Design review of the part built by this model. Coordinates are the model's own, in mm. Face numbers are marked on the shaded views. A direction names the side the tool comes from. Give positions to 0.01 mm unless a question says otherwise; leave off trailing zeros. Loops run counter-clockwise (first coordinate to the right, second up) from the corner with the lowest first, then second, coordinate; pieces in that order, holes last. Notation, with made-up numbers: M 3.25,-14 L 53.25,-14 A5 cw 53.25,-10 Z; hole C -7.75,88.5 d7. An arc over 180 degrees is marked long. Use a Markdown table: item, result. Add a question column.
(1) For the marked faces 1 and 2, list the 3-axis set-ups (+Z, -Z, +X, -X, +Y, -Y) from which the entire face can be reached by the end or side of a thin tool; tool diameter is ignored.
(2) Draft analysis for pull direction X (two halves, no side actions). For the marked faces 3, 4 and 5, state which applies: pulls with the +X half, pulls with the -X half, needs draft (parallel to the pull), parting line crosses it, or undercut.
(3) Add section A-A, the plane x = 1.25. Give the boundary of the cut face in (y, z).
(4) For probe 1 along Z at (x, y) = (2.25, 0); probe 2 along Y at (x, z) = (-4.5, 0); probe 3 along X at (y, z) = (5.75, -118.5), list the stretches that pass through material, from the lowest coordinate up.
(5) Add section B-B, the plane z = -104. Give the boundary of the cut face in (x, y).
(6) Add section C-C, the plane y = -7.5. Give the boundary of the cut face in (x, z), then the cut area to 3 significant figures.
(7) Add section D-D, the plane x = 10.75. Give the boundary of the cut face in (y, z).
(8) Insertion check: pin 1 Ø2 at (x, y) = (-10, -0.5) entering from -Z; pin 2 Ø2 at (x, y) = (5, 0.5) entering from -Z; pin 3 Ø5 at (x, y) = (-9, 8) entering from +Z (3 decimals); pin 4 Ø2 at (x, y) = (1, 8.5) entering from -Z. Each pin has a flat end and moves straight along its axis. Give the tip position at first contact, or say it passes through.
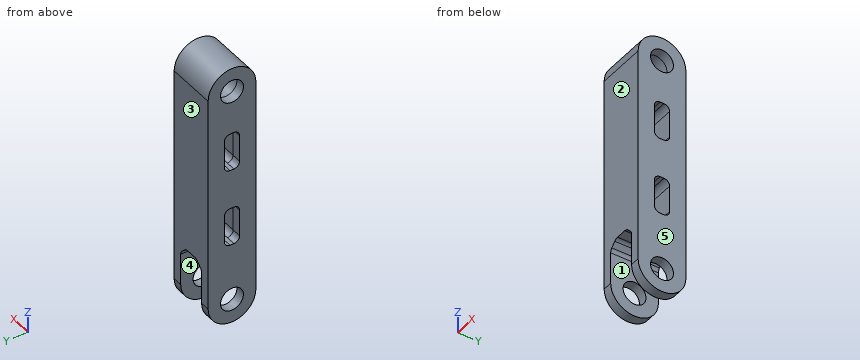
Autodesk Inventor part; units mm, degrees
ref_plane "YZ Plane" through (0, 0, 0) normal (1, 0, 0) x (0, 1, 0)
ref_plane "XZ Plane" through (0, 0, 0) normal (0, 1, 0) x (-1, 0, 0)
ref_plane "XY Plane" through (0, 0, 0) normal (0, 0, 1) x (1, 0, 0)
sketch "草圖1" plane through (0, 0, 0) normal (1, 0, 0) x (0, 1, 0)
  line L0 (0, 0) -> (0, -113.9)
  circle A0 centre (0, 0) radius 6
  circle A1 centre (0, -113.9) radius 6
  circle A2 centre (0, 0) radius 12.5
  circle A3 centre (0, -113.9) radius 12.5
  line L1 (12.5, 0) -> (12.5, -113.9)
  line L2 (-12.5, 0) -> (-12.5, -113.9)
  line L3 (4, -23) -> (-4, -23)
  line L4 (-4, -23) -> (-4, -43)
  line L5 (-4, -43) -> (4, -43)
  line L6 (4, -43) -> (4, -23)
  line L7 (4, -63.9) -> (-4, -63.9)
  line L8 (-4, -63.9) -> (-4, -83.9)
  line L9 (-4, -83.9) -> (4, -83.9)
  line L10 (4, -83.9) -> (4, -63.9)
  line L11 (12.5, -92) -> (-12.5, -92)
  point P0 (0, -23)
  point P1 (0, -63.9)
  dimension "d0" = 113.9
  dimension "d1" = 12
  dimension "d2" = 25
  dimension "d5" = 20
  dimension "d7" = 8
  dimension "d8" = 23
  dimension "d9" = 30
  dimension "d11" = 92
extrude "擠出1" add sketch "草圖1" along normal mid plane 16 contours A2 L1 L11 L0 L9 L10 L7 L5 L6 L3 | L0 L3 L4 L5 L7 L8 L9 L11 L2 A2 | A2
sketch "草圖4" plane through (8, 0, 0) normal (1, 0, 0) x (0, 0, -1)
  line L0 (63.9, -4) -> (63.9, 4)
  line L1 (63.9, 4) -> (83.9, 4)
  line L2 (83.9, 4) -> (83.9, -4)
  line L3 (83.9, -4) -> (63.9, -4)
  line L4 (43, 4) -> (43, -4)
  line L5 (43, -4) -> (23, -4)
  line L6 (23, -4) -> (23, 4)
  line L7 (23, 4) -> (43, 4)
  circle A0 centre (0, 0) radius 6
  line L8 (92, 12.5) -> (0, 12.5)
  arc A1 (0, 12.5) -> (0, -12.5) centre (0, 0) ccw
  line L9 (0, -12.5) -> (92, -12.5)
  line L10 (0, 12.5) -> (113.9, 12.5)
  line L11 (0, -12.5) -> (113.9, -12.5)
  circle A2 centre (113.9, 0) radius 12.5
  circle A3 centre (113.9, 0) radius 6
  point P0 (96, -12.5)
  point P1 (96, 12.5)
extrude "擠出4" add sketch "草圖4" along normal blind 5
sketch "草圖5" plane through (-8, 0, 0) normal (-1, 0, 0) x (0, 0, 1)
  line L0 (-92, -12.5) -> (0, -12.5)
  arc A0 (0, -12.5) -> (0, 12.5) centre (0, 0) ccw
  line L1 (0, 12.5) -> (-92, 12.5)
  circle A1 centre (0, 0) radius 6
  line L2 (-43, -4) -> (-43, 4)
  line L3 (-43, 4) -> (-23, 4)
  line L4 (-23, 4) -> (-23, -4)
  line L5 (-23, -4) -> (-43, -4)
  line L6 (-63.9, 4) -> (-63.9, -4)
  line L7 (-63.9, -4) -> (-83.9, -4)
  line L8 (-83.9, -4) -> (-83.9, 4)
  line L9 (-83.9, 4) -> (-63.9, 4)
  line L10 (0, -12.5) -> (-113.9, -12.5)
  line L11 (0, 12.5) -> (-113.9, 12.5)
  circle A2 centre (-113.9, 0) radius 12.5
  circle A3 centre (-113.9, 0) radius 6
extrude "擠出5" add sketch "草圖5" along normal blind 5
chamfer "倒角2" distance 4 angle 45 2 edges at (-8, 0, -92) (8, 0, -92)
fillet "圓角4" radius 3 4 edges at (-8, 0, -96) (-4, 0, -92) (4, 0, -92) (8, 0, -96)
fillet "圓角5" radius 3 8 edges at (0, 4, -23) (0, -4, -23) (0, -4, -43) (0, 4, -43) (0, 4, -63.9) (0, -4, -63.9) (0, -4, -83.9) (0, 4, -83.9)
properties part number "Link_OC" material "ABS 塑膠"
Established:
| question | item | result |
|---|---|---|
| 1 | face 1 | -Z, +Y, -Y |
| 1 | face 2 | +Z, -Z, +X, -X, -Y |
| 2 | face 3 | needs draft |
| 2 | face 4 | undercut |
| 2 | face 5 | pulls with the +X half |
| 3 | outline | M -12.5,-92 L 12.5,-92 L 12.5,0 A12.5 ccw -12.5,0 Z; hole C 0,0 d12; hole M -4,-80.9 A3 ccw -1,-83.9 L 1,-83.9 A3 ccw 4,-80.9 L 4,-66.9 A3 ccw 1,-63.9 L -1,-63.9 A3 ccw -4,-66.9 Z; hole M -4,-40 A3 ccw -1,-43 L 1,-43 A3 ccw 4,-40 L 4,-26 A3 ccw 1,-23 L -1,-23 A3 ccw -4,-26 Z |
| 4 | probe 1 | -92 to -83.9, -63.9 to -43, -23 to -6, 6 to 12.5 |
| 4 | probe 2 | -12.5 to -6, 6 to 12.5 |
| 4 | probe 3 | -13 to -8, 8 to 13 |
| 5 | outline | M -13,-12.5 L -8,-12.5 L -8,12.5 L -13,12.5 Z; M 8,-12.5 L 13,-12.5 L 13,12.5 L 8,12.5 Z |
| 6 | outline | M -13,-123.9 L -8,-123.9 L -8,-97.24 A3 cw -7.12,-95.12 L -4.88,-92.88 A3 cw -2.76,-92 L 2.76,-92 A3 cw 4.88,-92.88 L 7.12,-95.12 A3 cw 8,-97.24 L 8,-123.9 L 13,-123.9 L 13,10 L -13,10 Z |
| 6 | area | 2,990 mm^2 |
| 7 | outline | M -12.5,-113.9 A12.5 ccw 12.5,-113.9 L 12.5,0 A12.5 ccw -12.5,0 Z; hole C 0,-113.9 d12; hole C 0,0 d12; hole M -4,-80.9 A3 ccw -1,-83.9 L 1,-83.9 A3 ccw 4,-80.9 L 4,-66.9 A3 ccw 1,-63.9 L -1,-63.9 A3 ccw -4,-66.9 Z; hole M -4,-40 A3 ccw -1,-43 L 1,-43 A3 ccw 4,-40 L 4,-26 A3 ccw 1,-23 L -1,-23 A3 ccw -4,-26 Z |
| 8 | pin 1 | z = -126.4 |
| 8 | pin 2 | z = -94 |
| 8 | pin 3 | z = 11.225 |
| 8 | pin 4 | z = -92 |
